Input: part model. Units: mm. Frame: model coordinates. Coordinates: 2 decimals unless noted, no trailing zeros. Write each loop counter-clockwise with the first axis right and the second up, starting at its lowest first coordinate (ties: lowest second). Pieces come first, ordered by that corner, then holes.
1) Line query: L1, parallel to X at y = 2, z = 37.5; L2, parallel to Z at x = 501.5, y = 7.5. Output: solid intervals per line, ascending.
2) Section query B-B (z = 44). Output: boundary loops of the cut face in (x, y), then the cut area to 4 significant figures.
3) Section query A-A (y = 15.5). Output: boundary loops of the cut face in (x, z).
Autodesk Inventor part; units mm, degrees
ref_plane "YZ Plane" through (0, 0, 0) normal (1, 0, 0) x (0, 1, 0)
ref_plane "XZ Plane" through (0, 0, 0) normal (0, 1, 0) x (-1, 0, 0)
ref_plane "XY Plane" through (0, 0, 0) normal (0, 0, 1) x (1, 0, 0)
sketch "Sketch1" plane through (0, 0, 0) normal (0, 0, 1) x (1, 0, 0)
  line L0 (0, 0) -> (600, 0)
  line L1 (600, 0) -> (600, 18.55)
  line L2 (600, 18.55) -> (0, 18.55)
  line L3 (0, 18.55) -> (0, 0)
  dimension "d0" = 600
  dimension "d1" = 18.55
extrude "Extrusion1" add sketch "Sketch1" along normal blind 100
sketch "Sketch2" plane through (0, 18.55, 0) normal (0, 1, 0) x (1, 0, 0)
  line L0 (75, -31.45) -> (125, -31.45)
  line L1 (125, -31.45) -> (125, -68.55)
  line L2 (125, -68.55) -> (75, -68.55)
  line L3 (75, -68.55) -> (75, -31.45)
  line L4 (475, -31.45) -> (525, -31.45)
  line L5 (525, -31.45) -> (525, -68.55)
  line L6 (525, -68.55) -> (475, -68.55)
  line L7 (475, -68.55) -> (475, -31.45)
  line L8 (0, 0) -> (0, -100)
  line L9 (600, 0) -> (600, -100)
  line L10 (100, -31.45) -> (100, 0) construction
  line L11 (0, 0) -> (600, 0)
  line L12 (100, -68.55) -> (100, -100) construction
  line L13 (0, -100) -> (600, -100)
  dimension "d4" = 50
  dimension "d5" = 75
  dimension "d6" = 75
  dimension "d7" = 37.1
  dimension "d8" = 50
extrude "Extrusion2" cut sketch "Sketch2" against normal blind 100 contours L0 L1 L2 L3 | L4 L5 L6 L7
properties part number "table_bottont"
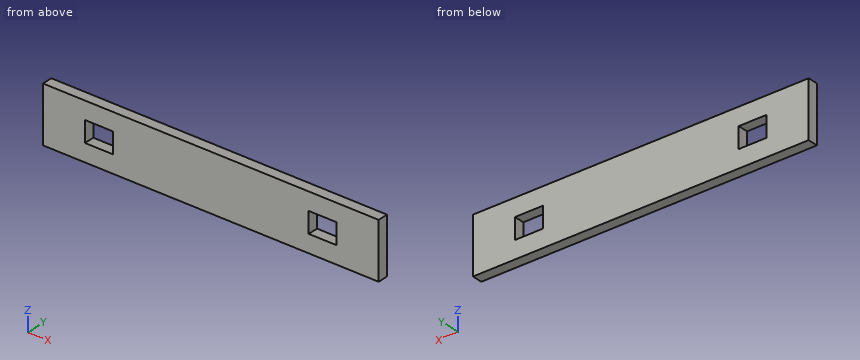
Answer:
1. L1: x = 0 to 75, 125 to 475, 525 to 600
1. L2: z = 0 to 31.45, 68.55 to 100
2. outline: (0, 0) - (75, 0) - (75, 18.55) - (0, 18.55) - close; (125, 0) - (475, 0) - (475, 18.55) - (125, 18.55) - close; (525, 0) - (600, 0) - (600, 18.55) - (525, 18.55) - close
2. area: 9,275 mm2
3. outline: (0, 0) - (600, 0) - (600, 100) - (0, 100) - close; hole (75, 31.45) - (125, 31.45) - (125, 68.55) - (75, 68.55) - close; hole (475, 31.45) - (525, 31.45) - (525, 68.55) - (475, 68.55) - close
